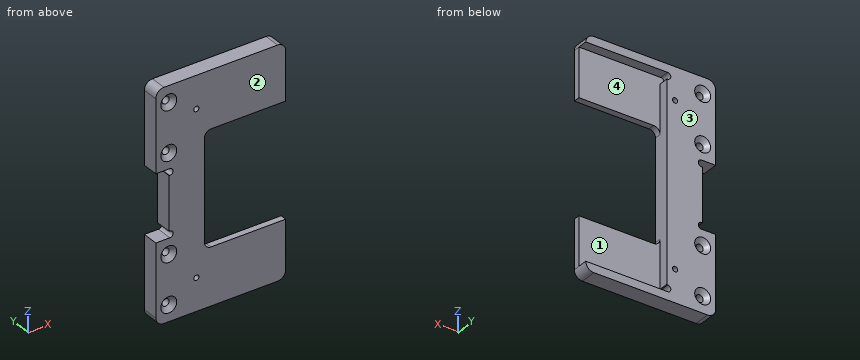
```python
from build123d import *

# Parameters (mm, degrees)
BOSS_EXTRUDE1_DEPTH                                 = 5
FILLET1_R                                           = 2
FILLET2_R                                           = 2.5
CUT_EXTRUDE2_REACH                                  = 7
CSK_FOR_M2_COUNTERSUNK_FLAT_HEAD_SCREW1_D           = 2.2
CSK_FOR_M2_COUNTERSUNK_FLAT_HEAD_SCREW1_DEPTH       = 5
CSK_FOR_M2_COUNTERSUNK_FLAT_HEAD_SCREW1_CSINK_D     = 4.9
CSK_FOR_M2_COUNTERSUNK_FLAT_HEAD_SCREW1_CSINK_ANGLE = 90
M2_TAPPED_HOLE1_D                                   = 1.6
M2_TAPPED_HOLE1_DEPTH                               = 5
SKETCH9_W                                           = 25.2
SKETCH9_H                                           = 12.5
CUT_EXTRUDE3_DEPTH                                  = 1.25
CUT_EXTRUDE4_DEPTH                                  = 1.25
SKETCH11_W                                          = 25
SKETCH11_H                                          = 4.5
CUT_EXTRUDE5_DEPTH                                  = 1.25
BOSS_EXTRUDE2_DEPTH                                 = 1.25
CUT_EXTRUDE6_DEPTH                                  = 1.75


with BuildPart() as part:
    # Sketch1 → Boss-Extrude1 (new body)
    with BuildSketch(Plane(origin=(0, 0, 0), x_dir=(1, 0, 0), z_dir=(0, 1, 0))):
        Polygon((0, 35), (0, 10.25), (4.1, 10.25), (4.1, -10.25), (0, -10.25), (0, -35), (40, -35), (40, -17.5), (15, -17.5), (15, 17.5), (40, 17.5), (40, 35), align=None)
    extrude(amount=BOSS_EXTRUDE1_DEPTH)

    # Fillet1
    fillet1_edges = [part.edges().sort_by_distance(p)[0] for p in [
        (15, 2.5, -17.5),
        (15, 2.5, 17.5),
    ]]
    fillet(fillet1_edges, radius=FILLET1_R)

    # Fillet2
    fillet2_edges = [part.edges().sort_by_distance(p)[0] for p in [
        (0, 2.5, -35),
        (40, 2.5, -35),
        (40, 2.5, 35),
        (0, 2.5, 35),
    ]]
    fillet(fillet2_edges, radius=FILLET2_R)

    # Sketch3 → Cut-Extrude2 (cut, up to next)
    with BuildSketch(Plane(origin=(0, 5, 0), x_dir=(1, 0, 0), z_dir=(0, 1, 0)), mode=Mode.PRIVATE) as cut_extrude2_sk1:
        with BuildLine():
            Line((4.1, 10.25), (4.35, 10.25))
            ThreePointArc((4.35, 10.25), (5.35, 9.25), (4.35, 8.25))
            Line((4.35, 8.25), (4.1, 8.25))
            Line((4.1, 8.25), (4.1, 10.25))
        make_face()
    cut_extrude2_tool1 = extrude(cut_extrude2_sk1.sketch, amount=-CUT_EXTRUDE2_REACH, mode=Mode.PRIVATE) & part.part
    add(cut_extrude2_tool1.solids().sort_by_distance((4.641756, 5, -9.25))[0], mode=Mode.SUBTRACT)
    # Sketch3 → Cut-Extrude2 (cut, up to next)
    with BuildSketch(Plane(origin=(0, 5, 0), x_dir=(1, 0, 0), z_dir=(0, 1, 0)), mode=Mode.PRIVATE) as cut_extrude2_sk2:
        with BuildLine():
            Line((4.1, -10.25), (4.1, -8.25))
            Line((4.1, -8.25), (4.35, -8.25))
            ThreePointArc((4.35, -8.25), (5.35, -9.25), (4.35, -10.25))
            Line((4.35, -10.25), (4.1, -10.25))
        make_face()
    cut_extrude2_tool2 = extrude(cut_extrude2_sk2.sketch, amount=-CUT_EXTRUDE2_REACH, mode=Mode.PRIVATE) & part.part
    add(cut_extrude2_tool2.solids().sort_by_distance((4.641756, 5, 9.25))[0], mode=Mode.SUBTRACT)

    # CSK for M2 Countersunk Flat Head Screw1
    with Locations(Plane(origin=(0, 5, 0), x_dir=(1, 0, 0), z_dir=(0, 1, 0))):
        with Locations((4, 30), (4, 15), (4, -15), (4, -30)):
            csk_for_m2_countersunk_flat_head_screw1 = CounterSinkHole(CSK_FOR_M2_COUNTERSUNK_FLAT_HEAD_SCREW1_D / 2, CSK_FOR_M2_COUNTERSUNK_FLAT_HEAD_SCREW1_CSINK_D / 2, depth=CSK_FOR_M2_COUNTERSUNK_FLAT_HEAD_SCREW1_DEPTH, counter_sink_angle=CSK_FOR_M2_COUNTERSUNK_FLAT_HEAD_SCREW1_CSINK_ANGLE)

    # M2 Tapped Hole1
    with Locations(Plane(origin=(0, 5, 0), x_dir=(1, 0, 0), z_dir=(0, 1, 0))):
        with Locations((12.5, -25), (12.5, 25)):
            Hole(M2_TAPPED_HOLE1_D / 2, depth=M2_TAPPED_HOLE1_DEPTH)

    # Sketch9 → Cut-Extrude3 (cut)
    with BuildSketch(Plane(origin=(0, 5, 0), x_dir=(1, 0, 0), z_dir=(0, 1, 0))):
        with Locations((27.4, 26.25)):
            Rectangle(SKETCH9_W, SKETCH9_H)
        with Locations((27.4, -26.25)):
            Rectangle(SKETCH9_W, SKETCH9_H)
    extrude(amount=-CUT_EXTRUDE3_DEPTH, mode=Mode.SUBTRACT)

    # Sketch10 → Cut-Extrude4 (cut)
    with BuildSketch(Plane(origin=(0, 5, 0), x_dir=(1, 0, 0), z_dir=(0, 1, 0))):
        with BuildLine():
            Line((14.8, 22), (14.8, 20))
            ThreePointArc((14.8, 20), (13.8, 21), (14.8, 22))
        make_face()
        with BuildLine():
            Line((14.8, 30.5), (14.8, 32.5))
            ThreePointArc((14.8, 32.5), (13.8, 31.5), (14.8, 30.5))
        make_face()
    cut_extrude4 = extrude(amount=-CUT_EXTRUDE4_DEPTH, mode=Mode.SUBTRACT)

    # Mirror1: CSK for M2 Countersunk Flat Head Screw1 across plane
    add(csk_for_m2_countersunk_flat_head_screw1.mirror(Plane(origin=(0, 2.5, 0), x_dir=(0, 0, 1), z_dir=(0, -1, 0))), mode=Mode.SUBTRACT)

    # Mirror2: Cut-Extrude4 across plane
    add(cut_extrude4.mirror(Plane.XY), mode=Mode.SUBTRACT)

    # Sketch11 → Cut-Extrude5 (cut)
    with BuildSketch(Plane(origin=(0, 5, 0), x_dir=(1, 0, 0), z_dir=(0, 1, 0))):
        with Locations((27.5, 17.75)):
            Rectangle(SKETCH11_W, SKETCH11_H)
        with Locations((27.5, -17.75)):
            Rectangle(SKETCH11_W, SKETCH11_H)
    extrude(amount=-CUT_EXTRUDE5_DEPTH, mode=Mode.SUBTRACT)

    # Sketch12 → Boss-Extrude2 (add)
    with BuildSketch(Plane(origin=(0, 3.75, 0), x_dir=(1, 0, 0), z_dir=(0, 1, 0))):
        with BuildLine():
            Line((14.8, 20), (15, 20))
            Line((15, 20), (15, 30.37258082))
            Line((15, 30.37258082), (14.8, 30.5))
            Line((14.8, 30.5), (14.8, 22))
            ThreePointArc((14.8, 22), (13.8, 21), (14.8, 20))
        make_face()
        with BuildLine():
            Line((14.8, -20), (15, -20))
            Line((15, -20), (15, -30.5))
            Line((15, -30.5), (14.8, -30.5))
            Line((14.8, -30.5), (14.8, -22))
            ThreePointArc((14.8, -22), (13.8, -21), (14.8, -20))
        make_face()
    extrude(amount=BOSS_EXTRUDE2_DEPTH)

    # Sketch13 → Cut-Extrude6 (cut)
    with BuildSketch(Plane(origin=(0, 3.75, 0), x_dir=(1, 0, 0), z_dir=(0, 1, 0))):
        with BuildLine():
            Line((14.8, 30.5), (15, 30.37258082))
            Line((15, 30.37258082), (15, 15.5))
            ThreePointArc((15, 15.5), (15.585786438, 16.914213562), (17, 17.5))
            Line((17, 17.5), (40, 17.5))
            Line((40, 17.5), (40, 32.5))
            Line((40, 32.5), (14.8, 32.5))
            ThreePointArc((14.8, 32.5), (13.8, 31.5), (14.8, 30.5))
        make_face()
        with BuildLine():
            Line((15, -15.5), (15, -30.5))
            Line((15, -30.5), (14.8, -30.5))
            ThreePointArc((14.8, -30.5), (13.8, -31.5), (14.8, -32.5))
            Line((14.8, -32.5), (40, -32.5))
            Line((40, -32.5), (40, -17.5))
            Line((40, -17.5), (17, -17.5))
            ThreePointArc((17, -17.5), (15.585786438, -16.914213562), (15, -15.5))
        make_face()
    extrude(amount=-CUT_EXTRUDE6_DEPTH, mode=Mode.SUBTRACT)


solid = part.part
```
Geometry check sheet. Reference: the model listing, model coordinates, mm. Face numbers are marked on the shaded views. A direction names the side the tool comes from. Round coordinates to 2 decimals unless told otherwise and drop trailing zeros. Write each loop counter-clockwise with the first axis right and the second up, starting at its lowest first coordinate (ties: lowest second). Pieces come first, ordered by that corner, then holes. Notation, with made-up numbers: (-16, -8.75) - (26, -8.75) arc R19 ccw to (26, 3.25) - close; hole circle Ø9 at (27.25, 40.5). An arc over 180 degrees is marked (long way). Write each question's results on one line, items separated by ' | '.
(1) Depth check by flat-ended pin: pin 1 Ø13.5 at (x, z) = (23, 22) entering from +Y; pin 2 Ø1.5 at (y, z) = (3, 4) entering from -X; pin 3 Ø1.8 at (x, z) = (4, -30) entering from -Y; pin 4 Ø3 at (x, z) = (4, -15) entering from +Y. Enter the tip coordinate at first touch or a pass-through.
Computed:
pin 1: stops at y = 2 | pin 2: stops at x = 4.1 | pin 3: passes through | pin 4: stops at y = 4.05
(2) Thickness scan on probe 1 along Z at (x, y) = (4, 2.3); probe 2 along Z at (x, y) = (12.5, 2.8); probe 3 along Z at (x, y) = (32, 0.4). Record the ranges inside material, lowest first. Write a range as from..to.
Computed:
probe 1: z = -35..-31.1, -28.9..-16.1, -13.9..-10.25, 10.25..13.9, 16.1..28.9, 31.1..35 | probe 2: z = -35..-25.8, -24.2..24.2, 25.8..35 | probe 3: z = -35..-17.5, 17.5..35
(3) Sectioned sample at B-B, the plane y = 2.9. Enter the section's corners in (x, z), plus the area to 3 significant figures.
Computed:
outline: (0, -32.5) arc R2.5 ccw to (2.5, -35) - (37.5, -35) arc R2.5 ccw to (40, -32.5) - (14.8, -32.5) arc R1 cw to (14.8, -30.5) - (15, -30.37) - (15, 30.5) - (14.8, 30.5) arc R1 cw to (14.8, 32.5) - (40, 32.5) arc R2.5 ccw to (37.5, 35) - (2.5, 35) arc R2.5 ccw to (0, 32.5) - (0, 10.25) - (4.35, 10.25) arc R1 cw to (4.35, 8.25) - (4.1, 8.25) - (4.1, -8.25) - (4.35, -8.25) arc R1 cw to (4.35, -10.25) - (0, -10.25) - close; hole circle Ø2.2 at (4, -30); hole circle Ø2.2 at (4, -15); hole circle Ø2.2 at (4, 15); hole circle Ø2.2 at (4, 30); hole circle Ø1.6 at (12.5, -25); hole circle Ø1.6 at (12.5, 25) | area: 1,060 mm^2
(4) Sectioned sample at D-D, the plane x = 12.5. Enter the section's corners in (y, z).
Computed:
outline: (0, -35) - (5, -35) - (5, -25.8) - (0, -25.8) - close; (0, -24.2) - (5, -24.2) - (5, 24.2) - (0, 24.2) - close; (0, 25.8) - (5, 25.8) - (5, 35) - (0, 35) - close
(5) Sectioned sample at A-A, the plane x = 22.5. Enter the section's corners in (y, z).
Computed:
outline: (0, -35) - (5, -35) - (5, -32.5) - (2, -32.5) - (2, -17.5) - (0, -17.5) - close; (0, 17.5) - (2, 17.5) - (2, 32.5) - (5, 32.5) - (5, 35) - (0, 35) - close
(6) Sectioned sample at C-C, the plane z = -25. Enter the section's corners in (x, y), plus the area to 3 significant figures.
Computed:
outline: (0, 0) - (11.7, 0) - (11.7, 5) - (0, 5) - close; (13.3, 0) - (40, 0) - (40, 2) - (15, 2) - (15, 5) - (13.3, 5) - close | area: 117 mm^2
(7) Draft check along Z on the marked faces 3 and 4. Enter one of: pulls with the +Z half, pulls with the -Z half, needs draft (parallel to the pull), parting line crosses it, or undercut.
Computed:
face 3: needs draft | face 4: undercut
(8) Set-up check for the marked faces 1 and 2: record each of +Z, -Z, +X, -X, +Y, -Y from which the full face is reachable in a straight line by a thin tool's end or side.
Computed:
face 1: +X, +Y | face 2: +Z, -Z, +X, -X, -Y
